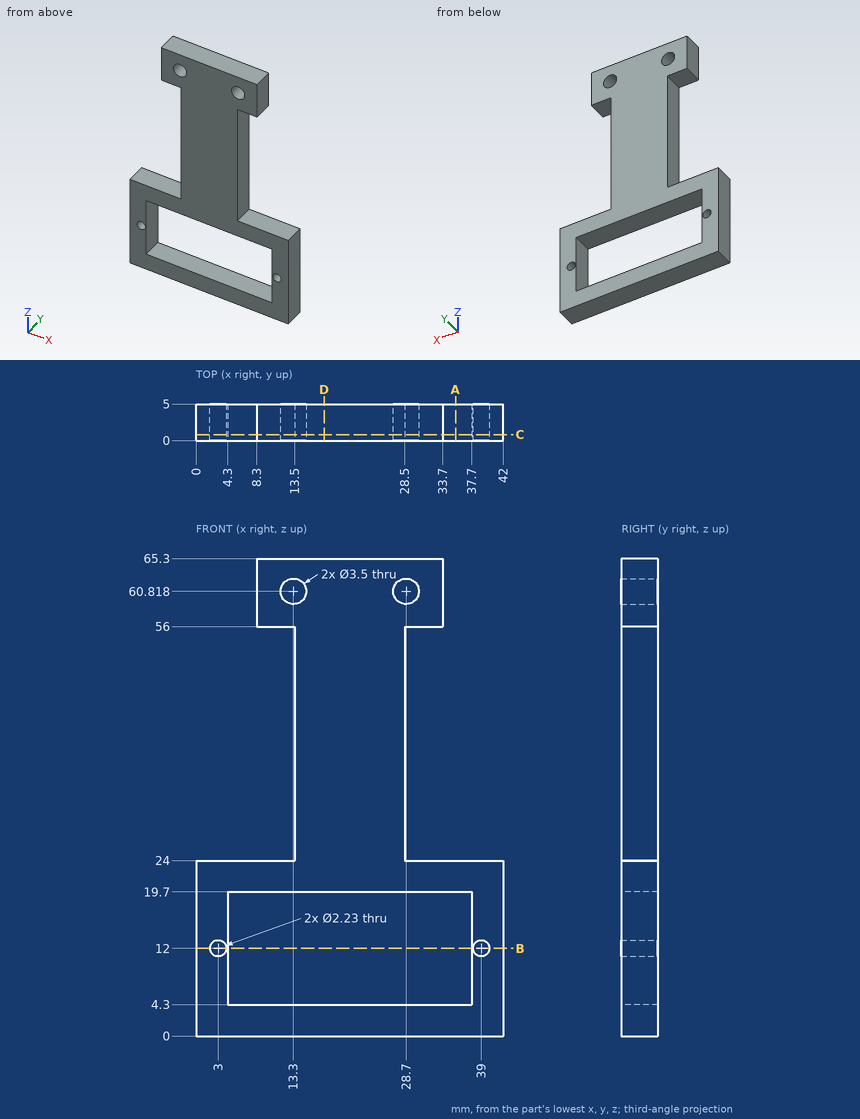
Design review of the part shown in the three views and the two pictorial views. Dimensions are in mm from the part's minimum x, y and z. Give positions to 0.01 mm unless a question says otherwise; leave off trailing zeros. Loops run counter-clockwise (first coordinate to the right, second up) from the corner with the lowest first, then second, coordinate; pieces in that order, holes last. Notation, with made-up numbers: (-1.75, 36.25) -> (11.25, 36.25) arc R31 cw to (11.25, 72.25) -> close; hole circle Ø4 at (51, 87.25). An arc over 180 degrees is marked (long way). Answer as a JSON object with one key per item and string values. Group by question number.
Q1. Insertion check: pin 1 (3 mm diameter, centred on y = 3, z = 30, fed in from -X); pin 2 (2 mm diameter, centred on y = 3, z = 34, fed in from +X); pin 3 (2.5 mm diameter, centred on y = 3, z = 63, fed in from -X). Each pin has a flat end and moves straight along its axis. Give the tip position at first contact, or say it passes through.
Q2. Take a section at A-A (x = 35.5). Write out the cut boundary in (y, z).
Q3. Take a section at B-B (z = 12). Write out the cut boundary in (x, y) (3 decimals), plus the area to 3 significant figures.
Q4. Wall thickness on line 1 along X through (y, z) = (2.15, 12) (3 decimals); line 2 along Z through (x, y) = (28.7, 1.4); line 3 along Z through (x, y) = (31, 4.6): over which ranges is each line inside the solid? List them lowest first.
Q5. Take a section at D-D (x = 17.5). Write out the cut boundary in (y, z).
Q6. Take a section at C-C (y = 0.8). State how many separate pieces and enclosed holes the cut face has, plus the area to 3 significant figures.
Answer below:
{
 "1": {"pin 1": "stops at x = 13.5", "pin 2": "stops at x = 28.5", "pin 3": "stops at x = 8.3"},
 "2": {"outline": "(0, 0) -> (5, 0) -> (5, 4.3) -> (0, 4.3) -> close; (0, 19.7) -> (5, 19.7) -> (5, 24) -> (0, 24) -> close"},
 "3": {"outline": "(0, 0) -> (1.885, 0) -> (1.885, 5) -> (0, 5) -> close; (4.115, 0) -> (4.3, 0) -> (4.3, 5) -> (4.115, 5) -> close; (37.7, 0) -> (37.885, 0) -> (37.885, 5) -> (37.7, 5) -> close; (40.115, 0) -> (42, 0) -> (42, 5) -> (40.115, 5) -> close", "area": "20.7 mm2"},
 "4": {"line 1": "x = 0 to 1.885, 4.115 to 4.3, 37.7 to 37.885, 40.115 to 42", "line 2": "z = 0 to 4.3, 19.7 to 24, 56 to 59.07, 62.57 to 65.3", "line 3": "z = 0 to 4.3, 19.7 to 24, 56 to 65.3"},
 "5": {"outline": "(0, 0) -> (5, 0) -> (5, 4.3) -> (0, 4.3) -> close; (0, 19.7) -> (5, 19.7) -> (5, 65.3) -> (0, 65.3) -> close"},
 "6": {"separate pieces": "1", "enclosed holes": "5", "area": "1,180 mm2"}
}
